The model under review builds one solid part; all positions refer to its coordinate system, in mm. A direction names the side the tool comes from. Round coordinates to 2 decimals unless told otherwise and drop trailing zeros. Order: outer loops, then holes, each group sorted by start corner. A loop starts at its lowest first (then second) coordinate and runs counter-clockwise, first axis right, second up.
```python
from build123d import *

# Parameters (mm, degrees)
SKETCH_R     = 4
PAD_DEPTH    = 8
SKETCH001_R  = 3.5
POCKET_DEPTH = 0.5
CHAMFER_SIZE = 0.5


with BuildPart() as part:
    # Sketch → Pad (new body)
    with BuildSketch(Plane.XY):
        with BuildLine():
            Line((-42.5, -10), (-27.5, -10))
            Line((-27.5, -10), (-27.5, -7))
            ThreePointArc((-25.5, -5), (-26.914214, -5.585786), (-27.5, -7))
            Line((-25.5, -5), (25.5, -5))
            ThreePointArc((27.5, -7), (26.914214, -5.585786), (25.5, -5))
            Line((27.5, -7), (27.5, -10))
            Line((27.5, -10), (42.5, -10))
            Line((42.5, -10), (42.5, 2))
            ThreePointArc((42.5, 2), (41.035534, 5.535534), (37.5, 7))
            Line((37.5, 7), (-37.5, 7))
            ThreePointArc((-37.5, 7), (-41.035534, 5.535534), (-42.5, 2))
            Line((-42.5, 2), (-42.5, -10))
        make_face()
        with Locations((-34.7, 0)):
            Circle(SKETCH_R, mode=Mode.SUBTRACT)
        with Locations((34.7, 0)):
            Circle(SKETCH_R, mode=Mode.SUBTRACT)
    extrude(amount=PAD_DEPTH)

    # Sketch001 (on Face2 of Pad) → Pocket (cut)
    with BuildSketch(Plane.XZ.offset(10)):
        with Locations((-35, 4)):
            Circle(SKETCH001_R)
        with Locations((35, 4)):
            Circle(SKETCH001_R)
    extrude(amount=-POCKET_DEPTH, mode=Mode.SUBTRACT)

    # Chamfer
    chamfer_edges = [part.edges().sort_by_distance(p)[0] for p in [
        (30.7, 0, 8),
        (-38.7, 0, 8),
    ]]
    chamfer(chamfer_edges, length=CHAMFER_SIZE)


solid = part.part
```
(1) Consider section D-D (x = 14). Write out the cut boundary in (y, z).
Data:
outline: (-5, 0) - (7, 0) - (7, 8) - (-5, 8) - close
(2) Draft analysis for pull direction Z (two halves, no side actions). For faces 4 (the cylindrical face through (-30.885, 1.201, 3.698)), 5 (the flat face through (-1, 1, 8)), 6 (the cylindrical face through (32.2, -9.8, 1.9)), state which applies: pulls with the +Z half, pulls with the -Z half, needs draft (parallel to the pull), parting line crosses it, or undercut.
Data:
face 4: needs draft
face 5: pulls with the +Z half
face 6: undercut
(3) Consider section C-C (x = -34.7). Write out the cut boundary in (y, z), and give its area (3 significant figures).
Data:
outline: (-10, 0) - (-4, 0) - (-4, 7.5) - (-4.5, 8) - (-10, 8) - (-10, 7.49) - (-9.5, 7.49) - (-9.5, 0.51) - (-10, 0.51) - close; (4, 0) - (7, 0) - (7, 8) - (4.5, 8) - (4, 7.5) - close
area: 68.3 mm2
(4) For faces 1 (the cylindrical face through (-26.9, -5.57, 3.94)), 2 (the flat face through (-35, -9.5, 4)), 3 (the flat face through (-42.5, -4, 4)), list the 3-axis set-ups (+Z, -Z, +X, -X, +Y, -Y) from which the entire face can be reached by the end or side of a thin tool; tool diameter is ignored.
Data:
face 1: +Z, -Z, -Y
face 2: -Y
face 3: +Z, -Z, -X, +Y, -Y
(5) Insertion check: pin 1 (6.5 mm diameter, centred on x = 34.7, y = 0, fed in from -Z); pin 2 (3.5 mm diameter, centred on x = 36.5, z = 4.5, fed in from -Y); pin 3 (2 mm diameter, centred on x = 17, z = 6.5, fed in from -Y). Each pin has a flat end and moves straight along its axis. Give the tip position at first contact, or say it passes through.
Data:
pin 1: passes through
pin 2: stops at y = -9.5
pin 3: stops at y = -5
(6) To check wall thickness, follow probe 1 along Y at (x, z) = (34.7, 1.75); probe 2 along X at (y, z) = (-1.75, 1.75); probe 3 along X at (y, z) = (0.5, 7.25). State the ranges of each line that lie inside material, in increasing order.
Data:
probe 1: y = -9.5 to -4, 4 to 7
probe 2: x = -42.5 to -38.3, -31.1 to 31.1, 38.3 to 42.5
probe 3: x = -42.5 to -38.67, -30.73 to 30.73, 38.67 to 42.5
(7) Consider section B-B (z = 2.5). Write out the cut boundary in (x, y).
Data:
outline: (-42.5, -10) - (-38.16, -10) - (-38.16, -9.5) - (-31.84, -9.5) - (-31.84, -10) - (-27.5, -10) - (-27.5, -7) arc R2 cw to (-25.5, -5) - (25.5, -5) arc R2 cw to (27.5, -7) - (27.5, -10) - (31.84, -10) - (31.84, -9.5) - (38.16, -9.5) - (38.16, -10) - (42.5, -10) - (42.5, 2) arc R5 ccw to (37.5, 7) - (-37.5, 7) arc R5 ccw to (-42.5, 2) - close; hole circle Ø8 at (-34.7, 0); hole circle Ø8 at (34.7, 0)
(8) Consider section A-A (y = 0). Write out the cut boundary in (x, z).
Data:
outline: (-42.5, 0) - (-38.7, 0) - (-38.7, 7.5) - (-39.2, 8) - (-42.5, 8) - close; (-30.7, 0) - (30.7, 0) - (30.7, 7.5) - (30.2, 8) - (-30.2, 8) - (-30.7, 7.5) - close; (38.7, 0) - (42.5, 0) - (42.5, 8) - (39.2, 8) - (38.7, 7.5) - close
